from build123d import *

# Parameters (mm, degrees)
SKETCH2_W           = 28
SKETCH2_H           = 28
SKETCH2_R           = 9.1
BOSS_EXTRUDE1_DEPTH = 5.2
BOSS_EXTRUDE2_START = -4
SKETCH2_4_W         = 28
SKETCH2_4_H         = 28
SKETCH2_4_R         = 9.1
BOSS_EXTRUDE2_DEPTH = 4
SKETCH3_R           = 2
CUT_EXTRUDE1_DEPTH  = 22.832086478
FILLET1_R           = 1


with BuildPart() as part:
    # Sketch2 → Boss-Extrude1 (new body)
    with BuildSketch(Plane(origin=(0, 0, 0), x_dir=(1, 0, 0), z_dir=(0, 1, 0))):
        Rectangle(SKETCH2_W, SKETCH2_H)
        with Locations(Location((0, 0, 0), (0, 0, 270))):
            Circle(SKETCH2_R, mode=Mode.SUBTRACT)
    extrude(amount=BOSS_EXTRUDE1_DEPTH)

    # Sketch2_4 → Boss-Extrude2 (add)
    # profile 1 of 2: a face of its own
    with BuildSketch(Plane(origin=(0, 0, 0), x_dir=(1, 0, 0), z_dir=(0, 1, 0)).offset(BOSS_EXTRUDE2_START)):
        Rectangle(SKETCH2_4_W, SKETCH2_4_H)
        with Locations(Location((0, 0, 0), (0, 0, 270))):
            Circle(SKETCH2_4_R, mode=Mode.SUBTRACT)
    # profile 2 of 2: a face of its own
    with BuildSketch(Plane(origin=(0, 0, 0), x_dir=(1, 0, 0), z_dir=(0, 1, 0)).offset(BOSS_EXTRUDE2_START)):
        with Locations(Location((0, 0, 0), (0, 0, 270))):
            Circle(SKETCH2_4_R)
    extrude(amount=BOSS_EXTRUDE2_DEPTH)

    # Sketch3 → Cut-Extrude1 (cut, through all)
    with BuildSketch(Plane(origin=(0, 5.2, 0), x_dir=(1, 0, 0), z_dir=(0, 1, 0))):
        with Locations(Location((10.217335854, -10.217335854, 0), (0, 0, 270))):
            Circle(SKETCH3_R)
        with Locations(Location((-10.217335854, -10.217335854, 0), (0, 0, 270))):
            Circle(SKETCH3_R)
        with Locations(Location((-10.217335854, 10.217335854, 0), (0, 0, 270))):
            Circle(SKETCH3_R)
        with Locations(Location((10.217335854, 10.217335854, 0), (0, 0, 270))):
            Circle(SKETCH3_R)
    extrude(amount=-CUT_EXTRUDE1_DEPTH, mode=Mode.SUBTRACT)

    # Fillet1
    fillet1_edges = [part.edges().sort_by_distance(p)[0] for p in [
        (10.217335854, -4, -12.217335854),
        (-10.217335854, -4, -12.217335854),
        (-10.217335854, -4, 8.217335854),
        (10.217335854, -4, 8.217335854),
    ]]
    fillet(fillet1_edges, radius=FILLET1_R)


solid = part.part
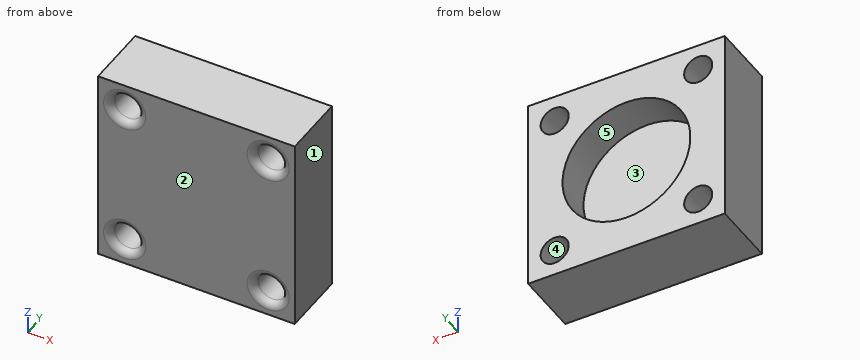
Model file for the job. Use its own axes, mm. Face numbers are marked on the shaded views. A direction names the side the tool comes from. Round coordinates to 2 decimals unless told otherwise and drop trailing zeros. Order: outer loops, then holes, each group sorted by start corner. A loop starts at its lowest first (then second) coordinate and runs counter-clockwise, first axis right, second up.
(1) Pin check, flat tip, straight feed: pin 1 (5.5 mm diameter, centred on x = 1, z = 2.5, fed in from +Y). Stop position of the tip, or through.
(2) Band-saw the part on B-B (y = 4.25). List the corners of the cut face in (x, z).
(3) Band-saw the part on C-C (z = 0). List the corners of the cut face in (x, y), then the cut area to 3 significant figures.
(4) Pull direction X, two halves, no side cores. Call the marked faces 1, 2 and 3: released by +X, released by -X, zero draft, split by the parting line, or undercut.
(5) 3-axis set-ups, long thin cutter, end or side, ignore diameter. For the marked faces 4 and 5: which of +Z, -Z, +X, -X, +Y, -Y reach the whole face in a straight line?
(6) Band-saw the part on D-D (y = -0.75). List the corners of the cut face in (x, z).
(7) Band-saw the part on A-A (x = 0). List the corners of the cut face in (y, z), then the cut area to 3 significant figures.
(8) Drill centre lines: line 1 (Z direction, x = -9, y = -2.5); line 2 (X direction, y = -2.5, z = -10); line 3 (Z direction, x = -8.5, y = -3.5). Where is each one in solid material? Low to high.
Verdict:
1. pin 1: stops at y = 0
2. outline: (-14, -14) - (14, -14) - (14, 14) - (-14, 14) - close; hole circle Ø4 at (-10.22, -10.22); hole circle Ø4 at (-10.22, 10.22); hole circle Ø18.2 at (0, 0); hole circle Ø4 at (10.22, -10.22); hole circle Ø4 at (10.22, 10.22)
3. outline: (-14, -4) - (14, -4) - (14, 5.2) - (9.1, 5.2) - (9.1, 0) - (-9.1, 0) - (-9.1, 5.2) - (-14, 5.2) - close
3. area: 163 mm2
4. face 1: released by +X
4. face 2: zero draft
4. face 3: undercut
5. face 4: +Y, -Y
5. face 5: +Y
6. outline: (-14, -14) - (14, -14) - (14, 14) - (-14, 14) - close; hole circle Ø4 at (-10.22, -10.22); hole circle Ø4 at (-10.22, 10.22); hole circle Ø4 at (10.22, -10.22); hole circle Ø4 at (10.22, 10.22)
7. outline: (-4, -14) - (5.2, -14) - (5.2, -9.1) - (0, -9.1) - (0, 9.1) - (5.2, 9.1) - (5.2, 14) - (-4, 14) - close
7. area: 163 mm2
8. line 1: z = -14 to -11.8, -8.63 to 8.63, 11.8 to 14
8. line 2: x = -14 to -12.21, -8.23 to 8.23, 12.21 to 14
8. line 3: z = -14 to -11.48, -8.95 to 8.95, 11.48 to 14
